For this review, take the finished solid that the model builds, in its own axes (mm). A direction names the side the tool comes from. Coordinates: 2 decimals unless noted, no trailing zeros. Order: outer loops, then holes, each group sorted by start corner. A loop starts at its lowest first (then second) coordinate and runs counter-clockwise, first axis right, second up. Notation, with made-up numbers: (12.25, 66) -> (46.25, 66) arc R20 cw to (46.25, 95) -> close; hole circle Ø2 at (46.25, 73). An arc over 180 degrees is marked (long way). Return JSON: item names as keys, results as strings. Group by question number.
Item 1: Draft analysis for pull direction Y (two halves, no side actions). For faces 1 (the cylindrical face through (72.384, -0.283, 7.43)), 2 (the flat face through (60, 0, 10)), 3 (the cylindrical face through (-0.987, 8.989, 0.752)), state which applies: +Y half, -Y half, draft (parallel to the pull), parting line (faces both ways), or undercut.
Item 2: Insertion check: pin 1 (1 mm diameter, centred on y = 9, z = 2, fed in from +X); pin 2 (5 mm diameter, centred on x = 58.5, y = -1.5, fed in from -Z); pin 3 (1.5 mm diameter, centred on x = 11.5, z = 13.5, fed in from +Y). Each pin has a flat end and moves straight along its axis. Give the tip position at first contact, or say it passes through.
Item 3: Take a section at A-A (z = 1.25). Write out the cut boundary in (x, y).
Item 4: Machinability: for faces 4 (the cylindrical face through (55.12, 1.5, 4.93)), 5 (the cylindrical face through (-0.985, 8.95, 14.287)), which of the approach directions +Z, -Z, +X, -X, +Y, -Y give a long, thin tool a straight path to every point of the face, cutting with its end or side? Answer none if there is none.
Item 5: For line 1 along X through (y, z) = (-0.5, 9); line 2 along Y through (x, z) = (-2.5, 5.75); line 3 along Z through (x, y) = (57, 0.5), list the stretches that pass through material, from the lowest coordinate up.
```python
from build123d import *

# Parameters (mm, degrees)
BOSS_EXTRUDE1_DEPTH = 15
SKETCH2_R           = 5
CUT_EXTRUDE1_DEPTH  = 10
FILLET1_R           = 2.5


with BuildPart() as part:
    # Sketch1 → Boss-Extrude1 (new body)
    with BuildSketch(Plane.XY):
        with BuildLine():
            ThreePointArc((-59.685185955, 6.992550832), (-52.362334802, 0), (-59.685185955, -6.992550832))
            Line((-59.685185955, -6.992550832), (59.311145469, -12.486697922))
            ThreePointArc((59.311145469, -12.486697922), (72.387665198, 1.24e-07), (59.311145222, 12.486697911))
            Line((59.311145222, 12.486697911), (-59.685185955, 6.992550832))
        make_face()
    extrude(amount=BOSS_EXTRUDE1_DEPTH)

    # Sketch2 → Cut-Extrude1 (cut)
    with BuildSketch(Plane(origin=(0, 0, 0), x_dir=(-1, 0, 0), z_dir=(0, 0, -1))):
        with Locations((-59.887665198, 0)):
            Circle(SKETCH2_R)
    extrude(amount=-CUT_EXTRUDE1_DEPTH, mode=Mode.SUBTRACT)

    # Fillet1
    fillet1_edges = [part.edges().sort_by_distance(p)[0] for p in [
        (72.387665198, 1.24e-07, 15),
        (-0.187020366, 9.739624371, 15),
        (-0.187020243, -9.739624377, 15),
        (-0.187020366, 9.739624371, 0),
        (72.387665198, 1.24e-07, 0),
        (-0.187020243, -9.739624377, 0),
    ]]
    fillet(fillet1_edges, radius=FILLET1_R)


solid = part.part
```
Findings below:
{
 "1": {"face 1": "parting line", "face 2": "undercut", "face 3": "+Y half"},
 "2": {"pin 1": "stops at x = 69", "pin 2": "stops at z = 10", "pin 3": "stops at y = 10.27"},
 "3": {"outline": "(-57.53, -6.76) -> (59.33, -12.15) arc R12.17 ccw (long way) to (59.33, 12.15) -> (-57.53, 6.76) arc R7 cw to start; hole circle Ø10 at (59.89, 0)"},
 "4": {"face 4": "-Z", "face 5": "+Z, -X, +Y"},
 "5": {"line 1": "x = -52.38 to 54.91, 64.86 to 72.38", "line 2": "y = -9.63 to 9.63", "line 3": "z = 10 to 15"}
}
